```python
from build123d import *

# Parameters (mm, degrees)
SKETCH1_R               = 35
BOSS_EXTRUDE1_DEPTH     = 10
SKETCH2_R               = 23.5
BOSS_EXTRUDE2_DEPTH     = 13
BOSS_EXTRUDE3_DEPTH     = 5
SKETCH5_R               = 1.5
CUT_EXTRUDE1_DEPTH      = 87.587143002
SKETCH9_W               = 4
SKETCH9_H               = 9
BOSS_EXTRUDE8_DEPTH     = 3
FILLET3_R               = 2
SKETCH11_R              = 10
CUT_EXTRUDE2_DEPTH      = 10
MIRROR2_COPY_1_SKETCH_R = 1.5
MIRROR2_COPY_1_DEPTH    = 87.587143002
FILLET3_OF_MIRROR2_R    = 2


with BuildPart() as part:
    # Sketch1 → Boss-Extrude1 (new body)
    with BuildSketch(Plane(origin=(0, 0, 0), x_dir=(0, 0, -1), z_dir=(1, 0, 0))):
        Circle(SKETCH1_R)
    extrude(amount=BOSS_EXTRUDE1_DEPTH)

    # Sketch2 → Boss-Extrude2 (add)
    with BuildSketch(Plane(origin=(10, 0, 0), x_dir=(0, 0, -1), z_dir=(1, 0, 0))):
        with Locations(Location((0, 0, 0), (0, 0, 180))):
            Circle(SKETCH2_R)
    extrude(amount=BOSS_EXTRUDE2_DEPTH)

    # Sketch4 → Boss-Extrude3 (add, symmetric)
    with BuildSketch(Plane(origin=(0, 13, 0), x_dir=(1, 0, 0), z_dir=(0, 1, 0))):
        Polygon((23, 35), (23, -35), (30.392057511, -43.809511096), (35.392057511, -43.809511096), (52.621859248, -23.275832977), (52.621859248, 23.275832977), (35.392057511, 43.809511096), (30.392057511, 43.809511096), align=None)
    boss_extrude3 = extrude(amount=BOSS_EXTRUDE3_DEPTH, both=True)

    # Sketch5 → Cut-Extrude1 (cut, through all)
    with BuildSketch(Plane(origin=(0, 18, 0), x_dir=(1, 0, 0), z_dir=(0, 1, 0))):
        with Locations(Location((32.892057511, -40.809511096, 0), (0, 0, 270))):
            Circle(SKETCH5_R)
    cut_extrude1 = extrude(amount=-CUT_EXTRUDE1_DEPTH, mode=Mode.SUBTRACT)

    # Mirror1: Cut-Extrude1 across plane
    add(cut_extrude1.mirror(Plane.XY), mode=Mode.SUBTRACT)

    # Sketch9 → Boss-Extrude8 (add)
    with BuildSketch(Plane(origin=(23, 0, 0), x_dir=(0, 0, -1), z_dir=(1, 0, 0))):
        with Locations((0, 22.5)):
            Rectangle(SKETCH9_W, SKETCH9_H)
    boss_extrude8 = extrude(amount=BOSS_EXTRUDE8_DEPTH)

    # Fillet3
    fillet3_edges = [part.edges().sort_by_distance(p)[0] for p in [
        (24.5, 27, -2),
        (24.5, 27, 2),
    ]]
    fillet(fillet3_edges, radius=FILLET3_R - 0.0001)  # a hair under: the kernel refuses the full size

    # Sketch11 → Cut-Extrude2 (cut)
    with BuildSketch(Plane.ZY):
        Circle(SKETCH11_R)
    extrude(amount=-CUT_EXTRUDE2_DEPTH, mode=Mode.SUBTRACT)

    # Mirror2: Boss-Extrude3, Cut-Extrude1, Boss-Extrude8 across plane
    add(boss_extrude3.mirror(Plane(origin=(0, -7, 0), x_dir=(0, 0, 1), z_dir=(0, -1, 0))))
    add(cut_extrude1.mirror(Plane(origin=(0, -7, 0), x_dir=(0, 0, 1), z_dir=(0, -1, 0))), mode=Mode.SUBTRACT)
    add(boss_extrude8.mirror(Plane(origin=(0, -7, 0), x_dir=(0, 0, 1), z_dir=(0, -1, 0))))

    # Mirror2 copy 1 sketch → Mirror2 copy 1 (cut, through all)
    with BuildSketch(Plane.XZ.offset(32)):
        with Locations(Location((32.892057511, -40.809511096, 0), (0, 0, 270))):
            Circle(MIRROR2_COPY_1_SKETCH_R)
    extrude(amount=-MIRROR2_COPY_1_DEPTH, mode=Mode.SUBTRACT)

    # Fillet3 of Mirror2
    fillet3_of_mirror2_edges = [part.edges().sort_by_distance(p)[0] for p in [
        (24.5, -41, -2),
        (24.5, -41, 2),
    ]]
    fillet(fillet3_of_mirror2_edges, radius=FILLET3_OF_MIRROR2_R - 0.0001)  # a hair under: the kernel refuses the full size


solid = part.part
```
Geometry: final body of the model. Coordinates: model frame, mm. A direction names the side the tool comes from. Coordinates: 2 decimals unless noted, no trailing zeros. Order: outer loops, then holes, each group sorted by start corner. A loop starts at its lowest first (then second) coordinate and runs counter-clockwise, first axis right, second up. Notation, with made-up numbers: M 83.25,32 L 90.25,32 A27 cw 90.25,60 Z; hole C 76,4.25 d1. An arc over 180 degrees is marked long. Answer in a Markdown table with one row per item. Add a question column.
Q1. Reachability of faces 1 (the flat face through (23, 13, 27)), 2 (the flat face through (23, -7, 0)), 3 (the flat face through (24, 21, -2)) from +Z, -Z, +X, -X, +Y, -Y: full face, straight path, thin tool, end or side. Return the list, or none.
Q2. Mould query, pull axis Y, two halves, no side actions, for faces 4 (the cylindrical face through (24.52, 26.43, -1.4)), 5 (the cylindrical face through (4.93, -9.76, -2.17)), 6 (the cylindrical face through (24.52, -40.43, -1.4)). Classes: released by +Y, released by -Y, zero draft, split by the parting line, or undercut.
Q3. Contact query for flat-ended pins moving along their axis: P1, Ø2.5, axis at x = 24.5, y = -36, coming from the +Z side; P2, Ø10, axis at x = 16.5, y = 18, coming from the +Z side; P3, Ø6, axis at y = 22.5, z = -25, coming from the +X side. Output: stop coordinate, or through.
Q4. Section query C-C on y = 11.5. Return the cut outline in (x, z), and give its area (3 significant figures).
Q5. Section query B-B on x = 42. Return the cut outline in (y, z), and give its area (3 significant figures).
Q6. Line query: L1, parallel to Y at x = 40, z = 4; L2, parallel to X at y = -22.5, z = 20; L3, parallel to X at y = -18.5, z = 9.5. Output: solid intervals per line, ascending.
Q7. Section query D-D on x = 8.5. Return the cut outline in (y, z), and give its area (3 significant figures).
Q8. Section query A-A on z = 13.5. Return the cut outline in (x, y).
Completed:
| question | item | result |
|---|---|---|
| 1 | face 1 | +Z, +Y |
| 1 | face 2 | +Z, -Z, +X |
| 1 | face 3 | -Z, +X, +Y |
| 2 | face 4 | released by +Y |
| 2 | face 5 | undercut |
| 2 | face 6 | released by -Y |
| 3 | P1 | stops at z = 2 |
| 3 | P2 | stops at z = 19.58 |
| 3 | P3 | stops at x = 10 |
| 4 | outline | M 0,-33.06 L 10,-33.06 L 10,-20.49 L 23,-20.49 L 23,-35 L 30.39,-43.81 L 35.39,-43.81 L 52.62,-23.28 L 52.62,23.28 L 35.39,43.81 L 30.39,43.81 L 23,35 L 23,20.49 L 10,20.49 L 10,33.06 L 0,33.06 Z; hole C 32.89,-40.81 d3; hole C 32.89,40.81 d3 |
| 4 | area | 3,360 mm2 |
| 5 | outline | M -32,-35.93 L -22,-35.93 L -22,35.93 L -32,35.93 Z; M 8,-35.93 L 18,-35.93 L 18,35.93 L 8,35.93 Z |
| 5 | area | 1,440 mm2 |
| 6 | L1 | y = -32 to -22, 8 to 18 |
| 6 | L2 | x = 0 to 10, 23 to 52.62 |
| 6 | L3 | x = 0 to 23 |
| 7 | outline | C 0,0 d70; hole C 0,0 d20 |
| 7 | area | 3,530 mm2 |
| 8 | outline | M 0,-32.29 L 10,-32.29 L 10,-19.24 L 23,-19.24 L 23,8 L 52.62,8 L 52.62,18 L 23,18 L 23,19.24 L 10,19.24 L 10,32.29 L 0,32.29 Z; M 23,-32 L 52.62,-32 L 52.62,-22 L 23,-22 Z |
